```python
from build123d import *

# Parameters (mm, degrees)
SKETCH1_R               = 38.5
SKETCH1_R_2             = 36.5
BOSS_EXTRUDE1_DEPTH     = 457.2
SKETCH2_R               = 1.95
CUT_EXTRUDE1_DEPTH      = 39.5
CUT_EXTRUDE1_DEPTH_BACK = 39.5
SKETCH3_R               = 1.95
CUT_EXTRUDE2_DEPTH      = 39.5000001
CUT_EXTRUDE2_DEPTH_BACK = 39.5000001


with BuildPart() as part:
    # Sketch1 → Boss-Extrude1 (new body)
    with BuildSketch(Plane(origin=(0, 0, 0), x_dir=(1, 0, 0), z_dir=(0, 1, 0))):
        Circle(SKETCH1_R)
        Circle(SKETCH1_R_2, mode=Mode.SUBTRACT)
    extrude(amount=BOSS_EXTRUDE1_DEPTH)

    # Sketch2 → Cut-Extrude1 (cut, two sides)
    with BuildSketch(Plane(origin=(0, 0, 0), x_dir=(0, 0, -1), z_dir=(1, 0, 0))) as cut_extrude1_sk:
        with Locations((0, 419.1)):
            Circle(SKETCH2_R)
    extrude(amount=CUT_EXTRUDE1_DEPTH, mode=Mode.SUBTRACT)
    extrude(cut_extrude1_sk.sketch, amount=-CUT_EXTRUDE1_DEPTH_BACK, mode=Mode.SUBTRACT)

    # Sketch3 → Cut-Extrude2 (cut, two sides)
    with BuildSketch(Plane.XY) as cut_extrude2_sk:
        with Locations((0, 419.1)):
            Circle(SKETCH3_R)
    extrude(amount=CUT_EXTRUDE2_DEPTH, mode=Mode.SUBTRACT)
    extrude(cut_extrude2_sk.sketch, amount=-CUT_EXTRUDE2_DEPTH_BACK, mode=Mode.SUBTRACT)


solid = part.part
```
Input: part model. Units: mm. Frame: model coordinates. Give positions to 0.01 mm unless a question says otherwise; leave off trailing zeros. Order: outer loops, then holes, each group sorted by start corner. A loop starts at its lowest first (then second) coordinate and runs counter-clockwise, first axis right, second up.
1. Cut plane A-A (z = -23). Return loops of the section in (x, y), and give its area (3 significant figures).
Computed:
outline: (-30.87, 0) - (-28.34, 0) - (-28.34, 457.2) - (-30.87, 457.2) - close; (28.34, 0) - (30.87, 0) - (30.87, 457.2) - (28.34, 457.2) - close
area: 2,320 mm2
2. Cut plane B-B (x = -16). Return loops of the section in (y, z).
Computed:
outline: (0, -35.02) - (457.2, -35.02) - (457.2, -32.81) - (0, -32.81) - close; (0, 32.81) - (457.2, 32.81) - (457.2, 35.02) - (0, 35.02) - close
3. Draft query along Z for faces 1 (the face through (-7.912, 225.4, 35.632)), 2 (the face through (-30.55, 225.4, 23.43)), 3 (the face through (23, 0, -29)). Return one class per face: released by +Z, released by -Z, zero draft, split by the parting line, or undercut.
Computed:
face 1: undercut
face 2: split by the parting line
face 3: zero draft
4. Cut plane C-C (y = 403.5). Return loops of the section in (x, z).
Computed:
outline: circle Ø77 at (0, 0); hole circle Ø73 at (0, 0)
5. Pin query (flat end, axial travel): pin 1 Ø2 at (y, z) = (59, -1.5) entering from -X; pin 2 Ø5 at (x, y) = (0, 419.1) entering from +Z; pin 3 Ø4 at (y, z) = (50.5, 18) entering from +X; pin 4 Ø12 at (y, z) = (78, -26) entering from +X. Return the tip coordinate at first contact, or that it passes through.
Computed:
pin 1: stops at x = -38.5
pin 2: stops at z = 38.5
pin 3: stops at x = 35.02
pin 4: stops at x = 32.9
6. Line query: probe 1 along X at (y, z) = (177, 0); probe 2 along Y at (x, z) = (37.95, 0); probe 3 along Z at (x, y) = (1.5, 76). Output: solid intervals per line, ascending.
Computed:
probe 1: x = -38.5 to -36.5, 36.5 to 38.5
probe 2: y = 0 to 417.15, 421.05 to 457.2
probe 3: z = -38.47 to -36.47, 36.47 to 38.47
